Build history of the part. All positions in model axes, mm. A direction names the side the tool comes from. Round coordinates to 2 decimals unless told otherwise and drop trailing zeros. Order: outer loops, then holes, each group sorted by start corner. A loop starts at its lowest first (then second) coordinate and runs counter-clockwise, first axis right, second up. Notation, with made-up numbers: (50.25, 12.25) -> (60.25, 12.25) arc R18 cw to (60.25, 43.25) -> close; hole circle Ø3 at (-10.5, 61.5). An arc over 180 degrees is marked (long way). Write item = value, one per line.
from build123d import *

# Parameters (mm, degrees)
SKETCH_1_W          = 28.5
SKETCH_1_H          = 28.5
SKETCH_1_R          = 2.75
EXTRUDE_1_DEPTH     = 11
SKETCH_2_W          = 6
SKETCH_2_H          = 0.8
SKETCH_2_W_2        = 0.8
SKETCH_2_H_2        = 6
EXTRUDE_2_DEPTH     = 12
SKETCH_3_R          = 1.5
SKETCH_3_R_2        = 2.15
SKETCH_3_W          = 1.2
SKETCH_3_H          = 3.3
SKETCH_3_H_2        = 3.309090331
CUT_EXTRUDE_1_DEPTH = 2
SKETCH_4_R          = 1.5
SKETCH_4_R_2        = 2.15
SKETCH_4_W          = 3.3
SKETCH_4_H          = 1.35
CUT_EXTRUDE_2_DEPTH = 20
CHAMFER_1_SIZE      = 1
CUT_EXTRUDE_3_DEPTH = 15


with BuildPart() as part:
    # Эскиз1 → Вытянуть1 (new body)
    with BuildSketch(Plane.XY):
        with Locations((14.25, 14.25)):
            Rectangle(SKETCH_1_W, SKETCH_1_H)
        with Locations((14.25, 14.25)):
            Circle(SKETCH_1_R, mode=Mode.SUBTRACT)
    extrude(amount=EXTRUDE_1_DEPTH)

    # Эскиз2 → Вытянуть2 (add)
    with BuildSketch(Plane.XY.offset(11)):
        with Locations((7.25, 6.25)):
            Rectangle(SKETCH_2_W, SKETCH_2_H)
        with Locations((21.25, 6.25)):
            Rectangle(SKETCH_2_W, SKETCH_2_H)
        with Locations((21.25, 22.25)):
            Rectangle(SKETCH_2_W_2, SKETCH_2_H_2)
        with Locations((7.25, 22.25)):
            Rectangle(SKETCH_2_W_2, SKETCH_2_H_2)
    extrude(amount=EXTRUDE_2_DEPTH)

    # Эскиз3 → Вырез-Вытянуть1 (cut)
    with BuildSketch(Plane.XZ.offset(-5.85)):
        with Locations((7.25, 16)):
            Circle(SKETCH_3_R)
        with Locations((21.25, 16)):
            Circle(SKETCH_3_R)
        with Locations((3.25, 19.75)):
            Circle(SKETCH_3_R_2)
        with Locations((11.25, 19.75)):
            Circle(SKETCH_3_R_2)
        with Locations((17.25, 19.764625166)):
            Circle(SKETCH_3_R_2)
        with Locations((25.25, 19.764625166)):
            Circle(SKETCH_3_R_2)
        with Locations((4.85, 12.65)):
            Rectangle(SKETCH_3_W, SKETCH_3_H)
        with Locations((9.65, 12.654545166)):
            Rectangle(SKETCH_3_W, SKETCH_3_H_2)
        with Locations((18.85, 12.654545166)):
            Rectangle(SKETCH_3_W, SKETCH_3_H_2)
        with Locations((23.65, 12.654545166)):
            Rectangle(SKETCH_3_W, SKETCH_3_H_2)
    extrude(amount=-CUT_EXTRUDE_1_DEPTH, mode=Mode.SUBTRACT)

    # Эскиз4 → Вырез-Вытянуть2 (cut)
    with BuildSketch(Plane.ZY.offset(-6.85)):
        with Locations(Location((16, 22.25, 0), (0, 0, 270))):
            Circle(SKETCH_4_R)
        with Locations((19.75, 18.25)):
            Circle(SKETCH_4_R_2)
        with Locations((19.75, 26.25)):
            Circle(SKETCH_4_R_2)
        with Locations((12.65, 24.575)):
            Rectangle(SKETCH_4_W, SKETCH_4_H)
        with Locations((12.65, 19.925)):
            Rectangle(SKETCH_4_W, SKETCH_4_H)
    extrude(amount=-CUT_EXTRUDE_2_DEPTH, mode=Mode.SUBTRACT)

    # Фаска1
    chamfer_1_edges = [part.edges().sort_by_distance(p)[0] for p in [
        (4.25, 6.25, 14.3),
        (4.25, 6.25, 23),
        (10.25, 6.25, 23),
        (10.25, 6.25, 14.309090331),
        (18.25, 6.25, 14.309090331),
        (18.25, 6.25, 23),
        (24.25, 6.25, 23),
        (24.25, 6.25, 14.309090331),
        (21.25, 25.25, 14.3),
        (21.25, 19.25, 14.3),
        (21.25, 19.25, 23),
        (21.25, 25.25, 23),
        (7.25, 25.25, 14.3),
        (7.25, 19.25, 14.3),
        (7.25, 19.25, 23),
        (7.25, 25.25, 23),
    ]]
    chamfer(chamfer_1_edges, length=CHAMFER_1_SIZE)

    # Эскиз5 → Вырез-Вытянуть3 (cut)
    with BuildSketch(Plane.XY.offset(11)):
        Polygon((3.927388562, 28.5), (0, 28.5), (0, 23.850233168), align=None)
    extrude(amount=-CUT_EXTRUDE_3_DEPTH, mode=Mode.SUBTRACT)


solid = part.part
Q1. Flat gauge pins, fed straight in: pin 1 (3 mm diameter, centred on y = 3.5, z = 15.5, fed in from -X); pin 2 (2 mm diameter, centred on x = 19.5, z = 13.5, fed in from +Y); pin 3 (6.5 mm diameter, centred on x = 20.5, z = 16.5, fed in from +Y); pin 4 (2.5 mm diameter, centred on x = 21.25, z = 16, fed in from -Y). Where does each tip first touch, or does it go through?
Check values:
pin_1 = through
pin_2 = 6.65
pin_3 = 25.25
pin_4 = 19.25
Q2. Probe probe 1 along Y at (x, z) = (14.25, 7.5); probe 2 along Z at (x, y) = (21.1, 22.25); probe 3 along Y at (x, z) = (7.5, 13.5). List the from-to ranges inside material, lowest first.
Check values:
probe_1 = 0 to 11.5, 17 to 28.5
probe_2 = 0 to 14.5, 17.5 to 23
probe_3 = 5.85 to 6.65, 20.6 to 23.9
Q3. Cut at D-D, the plane z = 3.75. List the corners of the cut face in (x, y).
Check values:
outline = (0, 0) -> (28.5, 0) -> (28.5, 28.5) -> (3.93, 28.5) -> (0, 23.85) -> close; hole circle Ø5.5 at (14.25, 14.25)
Q4. Mould opens along Z. For faces 1 (the face through (9.76, 6.24, 22.49)), 2 (the face through (7.2, 24.1, 19.7)), 3 (the face through (6.85, 22, 18)) say: released by +Z, released by -Z, zero draft, split by the parting line, or undercut.
Check values:
face_1 = released by +Z
face_2 = undercut
face_3 = zero draft
Q5. Cut at A-A, the plane x = 7.25. Give the number of separate pieces and of enclosed holes in the cut face, and give its area (3 significant figures).
Check values:
separate_pieces = 2
enclosed_holes = 1
area = 368 mm²
Q6. Cut at C-C, the plane y = 14.25. List the corners of the cut face in (x, z), and give its area (3 significant figures).
Check values:
outline = (0, 0) -> (11.5, 0) -> (11.5, 11) -> (0, 11) -> close; (17, 0) -> (28.5, 0) -> (28.5, 11) -> (17, 11) -> close
area = 253 mm²
Q7. Which spindle directions (+Z, -Z, +X, -X, +Y, -Y) get a long thin tool onto all of the face, cutting with end or side? Do faces 4 (the face through (21.65, 22, 18)), 5 (the face through (6.14, 6.24, 17.01)), 6 (the face through (7.2, 20.4, 19.8)), 7 (the face through (4.74, 6.24, 14.81)). Say none if no direction does.
Check values:
face_4 = +Z, +X, +Y
face_5 = -Y
face_6 = +X, -X
face_7 = -X, +Y, -Y
